Part model, mm, in its own coordinate system. A direction names the side the tool comes from. Round coordinates to 2 decimals unless told otherwise and drop trailing zeros. Write each loop counter-clockwise with the first axis right and the second up, starting at its lowest first coordinate (ties: lowest second). Pieces come first, ordered by that corner, then holes.
1) Drill centre lines: L1, parallel to X at y = -18.5, z = 5; L2, parallel to Z at x = -8, y = -15.5; L3, parallel to Z at x = -34.5, y = -20. Where is each one in solid material? Low to high.
2) Pull direction Z, two halves, no side cores. Call faces 4 (the flat face through (0, 0, -2)), 5 (the flat face through (0, -10, 16)), 6 (the flat face through (-18, -17, 10)): +Z half, -Z half, draft (parallel to the pull), parting line (faces both ways), or undercut.
3) Saw through at B-B on y = -12. Write the cut outline in (x, z).
4) Saw through at C-C on z = 12. Write the cut outline in (x, y) (3 decimals), and give its area (3 significant figures).
5) Saw through at A-A on x = -8. Write the cut outline in (y, z) (3 decimals), and give its area (3 significant figures).
6) Saw through at D-D on x = 1. Write the cut outline in (y, z), and give its area (3 significant figures).
7) Which spindle directions (+Z, -Z, +X, -X, +Y, -Y) get a long thin tool onto all of the face, cutting with end or side? Do faces 1 (the flat face through (-17, 3.2, 8)), 2 (the cylindrical face through (0.19, -9.75, 16.99)), 3 (the flat face through (-38.258, -20, 5)). Say none if no direction does.
8) Flat gauge pins, fed straight in: pin 1 (0.9 mm diameter, centred on x = -17, y = 0.5, fed in from +Z); pin 2 (1.7 mm diameter, centred on x = 16.5, z = 11, fed in from +Y); pin 3 (6.5 mm diameter, centred on x = -8, z = 5, fed in from +Y). Where does each tip first touch, or does it go through?
```python
from build123d import *

# Parameters (mm, degrees)
SKETCH1_R               = 16.175
BOSS_EXTRUDE1_DEPTH     = 2
BOSS_EXTRUDE2_DEPTH     = 16
BOSS_EXTRUDE3_DEPTH     = 2
BOSS_EXTRUDE4_DEPTH     = 10
SKETCH5_R               = 2.1
CUT_EXTRUDE3_DEPTH      = 10
CUT_EXTRUDE5_DEPTH      = 9
CUT_EXTRUDE5_DEPTH_BACK = 13


with BuildPart() as part:
    # Sketch1 → Boss-Extrude1 (new body)
    with BuildSketch(Plane.XY):
        Circle(SKETCH1_R)
        with BuildLine():
            ThreePointArc((17.382911868, 3.2), (0, 17.675), (-17.382911868, 3.2))
            Line((-17.382911868, 3.2), (-15.855302741, 3.2))
            ThreePointArc((-15.855302741, 3.2), (0, 16.175), (15.855302741, 3.2))
            Line((15.855302741, 3.2), (17.382911868, 3.2))
        make_face()
        with BuildLine():
            Line((-15.855302741, 3.2), (-17.382911868, 3.2))
            ThreePointArc((-17.382911868, 3.2), (-1.606651446, -17.6018265), (17.675, 0))
            ThreePointArc((17.675, 0), (17.6018265, 1.606651446), (17.382911868, 3.2))
            Line((17.382911868, 3.2), (15.855302741, 3.2))
            ThreePointArc((15.855302741, 3.2), (16.094877241, 1.607965045), (16.175, 0))
            ThreePointArc((16.175, 0), (-1.607965045, -16.094877241), (-15.855302741, 3.2))
        make_face()
    extrude(amount=-BOSS_EXTRUDE1_DEPTH)

    # Sketch1<4> → Boss-Extrude2 (add)
    with BuildSketch(Plane.XY):
        with BuildLine():
            Line((-15.855302741, 3.2), (-17.382911868, 3.2))
            ThreePointArc((-17.382911868, 3.2), (-1.606651446, -17.6018265), (17.675, 0))
            ThreePointArc((17.675, 0), (17.6018265, 1.606651446), (17.382911868, 3.2))
            Line((17.382911868, 3.2), (15.855302741, 3.2))
            ThreePointArc((15.855302741, 3.2), (16.094877241, 1.607965045), (16.175, 0))
            ThreePointArc((16.175, 0), (-1.607965045, -16.094877241), (-15.855302741, 3.2))
        make_face()
    extrude(amount=BOSS_EXTRUDE2_DEPTH)

    # Sketch2 → Boss-Extrude3 (add)
    with BuildSketch(Plane.XY.offset(16)):
        with BuildLine():
            Line((-9.580529002, -1.825), (-16.071714283, -1.825))
            ThreePointArc((-16.071714283, -1.825), (0, -16.175), (16.071714283, -1.825))
            Line((16.071714283, -1.825), (9.580529002, -1.825))
            ThreePointArc((9.580529002, -1.825), (0, -9.752802724), (-9.580529002, -1.825))
        make_face()
        with BuildLine():
            Line((-16.071714283, -1.825), (-17.580529002, -1.825))
            ThreePointArc((-17.580529002, -1.825), (0, -17.675), (17.580529002, -1.825))
            Line((17.580529002, -1.825), (16.071714283, -1.825))
            ThreePointArc((16.071714283, -1.825), (0, -16.175), (-16.071714283, -1.825))
        make_face()
    extrude(amount=BOSS_EXTRUDE3_DEPTH)

    # Sketch3 → Boss-Extrude4 (add)
    with BuildSketch(Plane.XY):
        with BuildLine():
            Line((-38.257911868, -17.675), (-17.382911868, 3.2))
            ThreePointArc((-17.382911868, 3.2), (-13.582445012, -11.310296747), (0, -17.675))
            Line((0, -17.675), (0, -22.675))
            Line((0, -22.675), (-38.257911868, -22.675))
            Line((-38.257911868, -22.675), (-38.257911868, -17.675))
        make_face()
    extrude(amount=BOSS_EXTRUDE4_DEPTH)

    # Sketch5 → Cut-Extrude3 (cut)
    with BuildSketch(Plane.XZ.offset(22.675)):
        with Locations((-30.257911868, 5)):
            Circle(SKETCH5_R)
        with Locations((-8, 5)):
            Circle(SKETCH5_R)
    extrude(amount=-CUT_EXTRUDE3_DEPTH, mode=Mode.SUBTRACT)

    # Sketch6 → Cut-Extrude5 (cut, two sides)
    with BuildSketch(Plane.XY.offset(10)) as cut_extrude5_sk:
        Polygon((-38.257911868, -17.675), (-22.582993568, -13.4749183), (-18.382911868, 2.2), align=None)
    extrude(amount=CUT_EXTRUDE5_DEPTH, mode=Mode.SUBTRACT)
    extrude(cut_extrude5_sk.sketch, amount=-CUT_EXTRUDE5_DEPTH_BACK, mode=Mode.SUBTRACT)


solid = part.part
```
Completed:
1. L1: x = -38.26 to -32.36, -28.16 to -10.1, -5.9 to 0
1. L2: z = -2 to 2.9, 7.1 to 18
1. L3: z = 0 to 10
2. face 4: -Z half
2. face 5: undercut
2. face 6: +Z half
3. outline: (-22.19, 0) - (-12.98, 0) - (-12.98, -2) - (12.98, -2) - (12.98, 18) - (-12.98, 18) - (-12.98, 10) - (-22.19, 10) - close; hole (-10.85, 0) - (10.85, 0) - (10.85, 16) - (-10.85, 16) - close
4. outline: (-17.383, 3.2) arc R17.675 ccw (long way) to (17.383, 3.2) - (15.855, 3.2) arc R16.175 cw (long way) to (-15.855, 3.2) - close
4. area: 89.4 mm2
5. outline: (-22.675, 0) - (-15.761, 0) - (-15.761, -2) - (15.761, -2) - (15.761, 0) - (-14.058, 0) - (-14.058, 2.9) - (-22.675, 2.9) - close; (-22.675, 7.1) - (-14.058, 7.1) - (-14.058, 16) - (-5.578, 16) - (-5.578, 18) - (-15.761, 18) - (-15.761, 10) - (-22.675, 10) - close
5. area: 144 mm2
6. outline: (-17.65, -2) - (17.65, -2) - (17.65, 0) - (-16.14, 0) - (-16.14, 16) - (-9.7, 16) - (-9.7, 18) - (-17.65, 18) - close
6. area: 111 mm2
7. face 1: +Z, +X, -X, +Y
7. face 2: +Z, +Y
7. face 3: +Z, -Z, -X, +Y, -Y
8. pin 1: stops at z = 16
8. pin 2: stops at y = 3.2
8. pin 3: stops at y = -11.62
